Design review of the part built by this model. Coordinates are the model's own, in mm. A direction names the side the tool comes from. Coordinates: 2 decimals unless noted, no trailing zeros. Write each loop counter-clockwise with the first axis right and the second up, starting at its lowest first coordinate (ties: lowest second). Pieces come first, ordered by that corner, then holes.
Q1. Take a section at D-D, the plane y = 65. Write out the cut boundary in (x, z).
Q2. For L1, parallel to Y at x = 0.4, z = -10; L2, parallel to X at y = 57.5, z = -15.5; L3, parallel to Z at x = 10.15, y = 35.5, list the stretches that pass through material, from the lowest coordinate up.
Q3. The part is to be moulded in two halves that separate along Y. For faces 1 (the flat face through (1, 35, -20)), 2 (the flat face through (13.38, 14.01, 2.49)), 3 (the flat face through (-10, 45, 3)), say which applies: released by +Y, released by -Y, zero draft, split by the parting line, or undercut.
Q4. For faces 4 (the flat face through (21, 15, 3)), 5 (the flat face through (-8, 19, 0)), 6 (the flat face through (13.38, 25.99, 2.49)), 7 (the flat face through (19, 50, 0)), 8 (the flat face through (2.6, 0, -7.5)), list the 3-axis set-ups (+Z, -Z, +X, -X, +Y, -Y) from which the entire face can be reached by the end or side of a thin tool; tool diameter is ignored.
Q5. Take a section at C-C, the plane x = -4. Write out the cut boundary in (y, z).
Q6. Take a section at A-A, the plane y = 50. Write out the cut boundary in (x, z).
Q7. For pin 1 Ø10 at (y, z) = (40, -11.5) entering from +X; pin 2 Ø3 at (y, z) = (35.5, -10) entering from -X; pin 3 Ø4 at (y, z) = (12.5, 1) entering from -X; pin 4 Ø12 at (x, y) = (-7.5, 25) entering from -Z, all flat-tipped, find the tip position at first contact; note any pin that passes through.
Q8. Take a section at B-B, the plane z = 2.75. State how many separate pieces and enclosed holes the cut face has, plus the area to 3 significant figures.
from build123d import *

# Parameters (mm, degrees)
BOSS_EXTRUDE1_DEPTH     = 70
CUT_EXTRUDE1_DEPTH      = 78.776388862
CUT_EXTRUDE1_DEPTH_BACK = 78.776388862
SKETCH2_R               = 2
SKETCH2_W               = 15
SKETCH2_H               = 15
SKETCH2_H_2             = 20
CUT_EXTRUDE2_DEPTH      = 79.217389371
CUT_EXTRUDE2_DEPTH_BACK = 79.217389371
SKETCH3_R               = 2
CHAMFER1_SIZE           = 2


with BuildPart() as part:
    # Sketch1 → Boss-Extrude1 (new body)
    with BuildSketch(Plane(origin=(0, 0, 0), x_dir=(1, 0, 0), z_dir=(0, 1, 0))):
        Polygon((-16.229090909, 0), (-1.229090909, 0), (-1.229090909, 20), (2.770909091, 20), (2.770909091, 0), (8.370909091, 0), (8.370909091, 20), (12.370909091, 20), (12.370909091, 0), (27.370909091, 0), (27.370909091, -5.261218749), (-16.229090909, -5.261218749), align=None)
    extrude(amount=BOSS_EXTRUDE1_DEPTH)

    # Sketch2 → Cut-Extrude1 (cut, two sides: drawn at the far end of the back side and taken through both)
    with BuildSketch(Plane(origin=(0, 0, 0), x_dir=(-1, 0, 0), z_dir=(0, 0, -1)).offset(-CUT_EXTRUDE1_DEPTH_BACK)):
        with Locations((-21.370909091, 50)):
            Circle(SKETCH2_R)
        with Locations(Location((10.229090909, 50, 0), (0, 0, 180))):
            Circle(SKETCH2_R)
        with Locations((10.229090909, 20)):
            Circle(SKETCH2_R)
        with Locations(Location((-21.370909091, 20, 0), (0, 0, 180))):
            Circle(SKETCH2_R)
        with Locations((-19.870909091, 62.5)):
            Rectangle(SKETCH2_W, SKETCH2_H)
        with Locations((-19.870909091, 35)):
            Rectangle(SKETCH2_W, SKETCH2_H_2)
        with Locations((8.729090909, 35)):
            Rectangle(SKETCH2_W, SKETCH2_H_2)
        with Locations((8.729090909, 62.5)):
            Rectangle(SKETCH2_W, SKETCH2_H)
        with Locations((8.729090909, 7.5)):
            Rectangle(SKETCH2_W, SKETCH2_H)
        with Locations((-19.870909091, 7.5)):
            Rectangle(SKETCH2_W, SKETCH2_H)
    extrude(amount=CUT_EXTRUDE1_DEPTH + CUT_EXTRUDE1_DEPTH_BACK, mode=Mode.SUBTRACT)

    # Sketch3 → Cut-Extrude2 (cut, two sides: drawn at the far end of the back side and taken through both)
    with BuildSketch(Plane(origin=(12.370909091, 0, 0), x_dir=(0, 0, -1), z_dir=(1, 0, 0)).offset(-CUT_EXTRUDE2_DEPTH_BACK)):
        with Locations((10, 57.5)):
            Circle(SKETCH3_R)
        with Locations((10, 35.5)):
            Circle(SKETCH3_R)
        with Locations((10, 13.5)):
            Circle(SKETCH3_R)
    extrude(amount=CUT_EXTRUDE2_DEPTH + CUT_EXTRUDE2_DEPTH_BACK, mode=Mode.SUBTRACT)

    # Chamfer1
    chamfer1_edges = [part.edges().sort_by_distance(p)[0] for p in [
        (-1.229090909, 25, 2.630609375),
        (12.370909091, 25, 2.630609375),
        (12.370909091, 45, 2.630609375),
        (12.370909091, 55, 2.630609375),
        (2.770909091, 35, 0),
        (8.370909091, 35, 0),
        (12.370909091, 50, 0),
        (12.370909091, 20, 0),
        (-1.229090909, 50, 0),
        (-1.229090909, 20, 0),
        (12.370909091, 15, 2.630609375),
        (-1.229090909, 15, 2.630609375),
        (-1.229090909, 55, 2.630609375),
        (-1.229090909, 45, 2.630609375),
    ]]
    chamfer(chamfer1_edges, length=CHAMFER1_SIZE)


solid = part.part
Responses:
1. outline: (-1.23, -20) - (2.77, -20) - (2.77, -2) - (4.77, 0) - (6.37, 0) - (8.37, -2) - (8.37, -20) - (12.37, -20) - (12.37, 5.26) - (-1.23, 5.26) - close
2. L1: y = 0 to 11.5, 15.5 to 33.5, 37.5 to 55.5, 59.5 to 70
2. L2: x = -1.23 to 2.77, 8.37 to 12.37
2. L3: z = -20 to -12, -8 to 5.26
3. face 1: zero draft
3. face 2: released by -Y
3. face 3: undercut
4. face 4: +Z, -Z, +X, -Y
4. face 5: -Z, -X, +Y, -Y
4. face 6: +Z, -Z, +X
4. face 7: -Z, +X, +Y, -Y
4. face 8: +Z, -Z, +X, -X, -Y
5. outline: (15, 0) - (25, 0) - (25, 5.26) - (15, 5.26) - close; (45, 0) - (55, 0) - (55, 5.26) - (45, 5.26) - close
6. outline: (-16.23, 0) - (-12.23, 0) - (-12.23, 5.26) - (-16.23, 5.26) - close; (-8.23, 0) - (-3.23, 0) - (-1.23, -2) - (-1.23, -20) - (2.77, -20) - (2.77, -2) - (4.77, 0) - (6.37, 0) - (8.37, -2) - (8.37, -20) - (12.37, -20) - (12.37, -2) - (14.37, 0) - (19.37, 0) - (19.37, 5.26) - (-8.23, 5.26) - close; (23.37, 0) - (27.37, 0) - (27.37, 5.26) - (23.37, 5.26) - close
7. pin 1: stops at x = 12.37
7. pin 2: passes through
7. pin 3: stops at x = -2.73
7. pin 4: stops at z = -1.73
8. separate pieces: 1
8. enclosed holes: 4
8. area: 1,520 mm2
